Autodesk Inventor part; units mm, degrees
ref_plane "YZ Plane" through (0, 0, 0) normal (1, 0, 0) x (0, 1, 0)
ref_plane "XZ Plane" through (0, 0, 0) normal (0, 1, 0) x (-1, 0, 0)
ref_plane "XY Plane" through (0, 0, 0) normal (0, 0, 1) x (1, 0, 0)
sketch "Sketch1" plane through (0, 0, 0) normal (0, 0, 1) x (1, 0, 0)
  line L0 (-12.1708, 16.0073) -> (13.2292, 16.0073)
  line L1 (13.2292, 16.0073) -> (13.2292, -34.7927)
  line L2 (13.2292, -34.7927) -> (-12.1708, -34.7927)
  line L3 (-12.1708, -34.7927) -> (-12.1708, 16.0073)
  line L4 (11.9592, 14.7373) -> (-10.9008, 14.7373)
  line L5 (-10.9008, 14.7373) -> (-10.9008, -33.5227)
  line L6 (-10.9008, -33.5227) -> (11.9592, -33.5227)
  line L7 (11.9592, -33.5227) -> (11.9592, 14.7373)
  point P0 (0, 0)
  dimension "d0" = 25.4
  dimension "d1" = 50.8
  dimension "d2" = 1.27
extrude "Extrusion1" add sketch "Sketch1" along normal blind 374.65
sketch "Sketch2" plane through (-12.1708, 16.0073, 0) normal (0, 1, 0) x (1, 0, 0)
  circle A0 centre (12.7, -12.7) radius 1.7272
  line L0 (25.4, 0) -> (0, 0)
  line L1 (0, 0) -> (0, -374.65)
  point P0 (12.1708, 0)
  dimension "d5" = 3.4544
  dimension "d6" = 12.7
  dimension "d7" = 12.7
extrude "Extrusion2" cut sketch "Sketch2" against normal through all
pattern_linear "Rectangular Pattern1" count 37 spacing 25.4 along (0, 0, 1) of "Extrusion2"
sketch "Sketch5" plane through (13.2292, -34.7927, 0) normal (1, 0, 0) x (0, 0, -1)
  circle A0 centre (-347.6625, 25.4) radius 14.2875
  line L0 (-374.65, 0) -> (-374.65, 50.8)
  line L1 (0, 50.8) -> (-374.65, 50.8)
  circle A1 centre (-225.425, 25.4) radius 14.2875
  circle A2 centre (-28.575, 25.4) radius 14.2875
  circle A3 centre (-119.0625, 25.4) radius 14.2875
  point P0 (0, 34.7927)
  dimension "d46" = 28.575
  dimension "d48" = 25.4
  dimension "d49" = 28.575
  dimension "d50" = 149.225
  dimension "d51" = 25.4
  dimension "d52" = 28.575
  dimension "d54" = 25.4
  dimension "d57" = 346.075
  dimension "d58" = 28.575
  dimension "d59" = 241.3
  dimension "d60" = 25.4
  dimension "d61" = 12.7
extrude "Extrusion5" cut sketch "Sketch5" against normal through all
equation "\"d3\" = d13"
equation "\"d10\" = d14"
equation "\"d13\" = 374.65"
equation "\"d14\" = d13"
equation "\"d32\" = 101.6"
properties part number "AIntakeVersa"
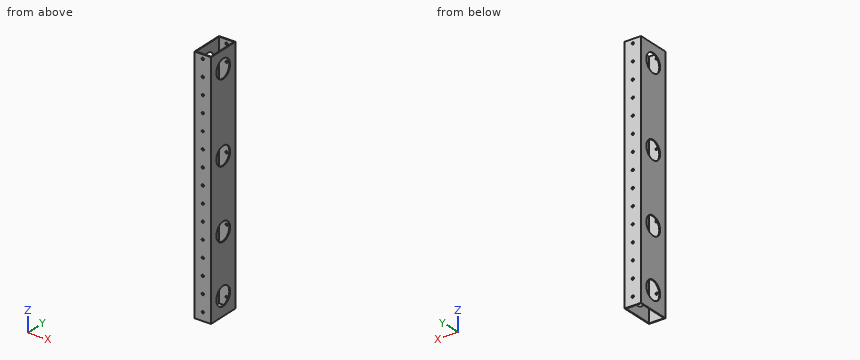
CAD build for the part. Positions are in the model's coordinates, mm. Round coordinates to 2 decimals unless told otherwise and drop trailing zeros. Loops run counter-clockwise (first coordinate to the right, second up) from the corner with the lowest first, then second, coordinate; pieces in that order, holes last. Notation, with made-up numbers: M 53,59 L 110,59 A25 ccw 110,74 Z; hole C 73,-39 d7. An arc over 180 degrees is marked long. Return JSON: item names as keys, results as strings. Group by question number.
(1) Saw through at C-C, the plane z = 232. List the corners of the cut face in (x, y), and give its area (3 significant figures).
(2) Saw through at B-B, the plane x = 7.5. List the corners of the cut face in (y, z).
(3) Wall check: probe 1 along Y at (x, z) = (5.25, 206); probe 2 along X at (y, z) = (-34, 114); probe 3 along X at (y, z) = (2, 173.5). Give the ranges that are in metal, low to high. Write a range as [from, to].
(4) Saw through at A-A, the plane z = 284.5. List the corners of the cut face in (x, y).
Answer list:
{
 "1": {"outline": "M -12.17,-34.79 L 13.23,-34.79 L 13.23,-22.08 L 11.96,-22.08 L 11.96,-33.52 L -10.9,-33.52 L -10.9,-22.08 L -12.17,-22.08 Z; M -12.17,3.29 L -10.9,3.29 L -10.9,14.74 L 11.96,14.74 L 11.96,3.29 L 13.23,3.29 L 13.23,16.01 L -12.17,16.01 Z", "area": "123 mm2"},
 "2": {"outline": "M -34.79,0 L -33.52,0 L -33.52,374.65 L -34.79,374.65 Z; M 14.74,0 L 16.01,0 L 16.01,374.65 L 14.74,374.65 Z"},
 "3": {"probe 1": "[-34.79, -33.52], [14.74, 16.01]", "probe 2": "[-12.17, -1.17], [2.23, 13.23]", "probe 3": "[-12.17, -10.9], [11.96, 13.23]"},
 "4": {"outline": "M -12.17,-34.79 L 13.23,-34.79 L 13.23,16.01 L -12.17,16.01 Z; hole M -10.9,-33.52 L 11.96,-33.52 L 11.96,14.74 L -10.9,14.74 Z"}
}
